Design review of the part built by this model. Coordinates are the model's own, in mm. A direction names the side the tool comes from. Give positions to 0.01 mm unless a question says otherwise; leave off trailing zeros. Loops run counter-clockwise (first coordinate to the right, second up) from the corner with the lowest first, then second, coordinate; pieces in that order, holes last.
from build123d import *

# Parameters (mm, degrees)
SKETCH1_R           = 1.651
BOSS_EXTRUDE1_DEPTH = 6.35
SKETCH2_W           = 12.7
SKETCH2_H           = 3.175
CUT_EXTRUDE7_DEPTH  = 8.89
FILLET2_R           = 1.27
SKETCH4_W           = 3.175
SKETCH4_H           = 19.05
CUT_EXTRUDE8_DEPTH  = 192.82600491
FILLET3_R           = 1.27
SKETCH5_R           = 3.175
CUT_EXTRUDE9_DEPTH  = 2.54


with BuildPart() as part:
    # Sketch1 → Boss-Extrude1 (new body)
    with BuildSketch(Plane(origin=(0, 0, 0), x_dir=(1, 0, 0), z_dir=(0, 1, 0))):
        Polygon((75.155177047, 61.997896552), (75.155177047, 11.997896552), (91.919177047, 11.997896552), (91.919177047, 20.379896552), (83.537177047, 20.379896552), (83.537177047, 53.615896552), (173.037829354, 53.615896552), (173.037829354, 20.379896552), (164.655829354, 20.379896552), (164.655829354, 11.997896552), (181.419829354, 11.997896552), (181.419829354, 61.997896552), align=None)
        with Locations(Location((80.3721812, 16.064784874, 0), (0, 0, 270))):
            Circle(SKETCH1_R, mode=Mode.SUBTRACT)
        with Locations(Location((80.3721812, 57.93100823, 0), (0, 0, 270))):
            Circle(SKETCH1_R, mode=Mode.SUBTRACT)
        with Locations(Location((88.7874552, 16.064784874, 0), (0, 0, 270))):
            Circle(SKETCH1_R, mode=Mode.SUBTRACT)
        with Locations(Location((167.7875512, 57.93100823, 0), (0, 0, 270))):
            Circle(SKETCH1_R, mode=Mode.SUBTRACT)
        with Locations(Location((88.7874552, 57.93100823, 0), (0, 0, 270))):
            Circle(SKETCH1_R, mode=Mode.SUBTRACT)
        with Locations(Location((176.2028252, 57.93100823, 0), (0, 0, 270))):
            Circle(SKETCH1_R, mode=Mode.SUBTRACT)
        with Locations(Location((176.2028252, 16.064784874, 0), (0, 0, 270))):
            Circle(SKETCH1_R, mode=Mode.SUBTRACT)
        with Locations(Location((167.7875512, 16.064784874, 0), (0, 0, 270))):
            Circle(SKETCH1_R, mode=Mode.SUBTRACT)
    extrude(amount=BOSS_EXTRUDE1_DEPTH)

    # Sketch2 → Cut-Extrude7 (cut)
    with BuildSketch(Plane(origin=(181.419829354, 0, 0), x_dir=(0, 0, -1), z_dir=(1, 0, 0))):
        with Locations((43.747896552, 4.7625)):
            Rectangle(SKETCH2_W, SKETCH2_H)
    extrude(amount=-CUT_EXTRUDE7_DEPTH, mode=Mode.SUBTRACT)

    # Fillet2
    fillet2_edges = [part.edges().sort_by_distance(p)[0] for p in [
        (177.228829354, 6.35, -37.397896552),
        (177.228829354, 6.35, -50.097896552),
        (177.228829354, 3.175, -50.097896552),
        (177.228829354, 3.175, -37.397896552),
    ]]
    fillet(fillet2_edges, radius=FILLET2_R)

    # Sketch4 → Cut-Extrude8 (cut, through all)
    with BuildSketch(Plane(origin=(0, 6.35, 0), x_dir=(1, 0, 0), z_dir=(0, 1, 0))):
        with Locations((81.949677047, 29.904896552)):
            Rectangle(SKETCH4_W, SKETCH4_H)
    extrude(amount=-CUT_EXTRUDE8_DEPTH, mode=Mode.SUBTRACT)

    # Fillet3
    fillet3_edges = [part.edges().sort_by_distance(p)[0] for p in [
        (83.537177047, 3.175, -39.429896552),
        (80.362177047, 3.175, -20.379896552),
        (80.362177047, 3.175, -39.429896552),
    ]]
    fillet(fillet3_edges, radius=FILLET3_R)

    # Sketch5 → Cut-Extrude9 (cut)
    with BuildSketch(Plane.XZ):
        with Locations((88.7874552, -16.064784874)):
            Circle(SKETCH5_R)
        with Locations(Location((88.7874552, -57.93100823, 0), (0, 0, 270))):
            Circle(SKETCH5_R)
        with Locations(Location((167.7875512, -57.93100823, 0), (0, 0, 270))):
            Circle(SKETCH5_R)
        with Locations((167.7875512, -16.064784874)):
            Circle(SKETCH5_R)
    extrude(amount=-CUT_EXTRUDE9_DEPTH, mode=Mode.SUBTRACT)


solid = part.part
Q1. Take a section at C-C (y = 1.25). Give the boundary of the cut face in (x, z) (3 decimals).
Results:
outline: (75.155, -61.998) - (181.42, -61.998) - (181.42, -11.998) - (164.656, -11.998) - (164.656, -15.542) arc R3.175 cw (long way) to (164.656, -16.587) - (164.656, -20.38) - (173.038, -20.38) - (173.038, -53.616) - (83.537, -53.616) - (83.537, -40.7) arc R1.27 ccw to (82.267, -39.43) - (81.632, -39.43) arc R1.27 cw to (80.362, -38.16) - (80.362, -21.65) arc R1.27 cw to (81.632, -20.38) - (91.919, -20.38) - (91.919, -16.587) arc R3.175 cw (long way) to (91.919, -15.542) - (91.919, -11.998) - (75.155, -11.998) - close; hole circle Ø3.302 at (80.372, -57.931); hole circle Ø3.302 at (80.372, -16.065); hole circle Ø6.35 at (88.787, -57.931); hole circle Ø6.35 at (167.788, -57.931); hole circle Ø3.302 at (176.203, -57.931); hole circle Ø3.302 at (176.203, -16.065)
Q2. Draft analysis for pull direction Z (two halves, no side actions). For faces 1 (the face through (173, 3, -11.998)), 2 (the face through (129, 3, -61.998)), 3 (the face through (170.96, 1.25, -16.2)), 4 (the face through (91.919, 3, -16)), state which applies: pulls with the +Z half, pulls with the -Z half, needs draft (parallel to the pull), parting line crosses it, or undercut.
Results:
face 1: pulls with the +Z half
face 2: pulls with the -Z half
face 3: undercut
face 4: needs draft
Q3. Take a section at D-D (x = 125.5). Give the boundary of the cut face in (y, z).
Results:
outline: (0, -62) - (6.35, -62) - (6.35, -53.62) - (0, -53.62) - close
Q4. Tool access review of faces 5 (the face through (128, 3, -53.616)), 6 (the face through (177, 3.175, -44)), 7 (the face through (166, 2.54, -59)): name each direction out of +Z, -Z, +X, -X, +Y, -Y from which nothing blocks a thin tool from reaching the whole face with its end or side.
Results:
face 5: +Y, -Y
face 6: +X, +Y
face 7: -Y
Q5. Insertion check: pin 1 (2 mm diameter, centred on x = 176.2, z = -57.93, fed in from +Y); pin 2 (9 mm diameter, centred on x = 177, z = -44.5, fed in from +Y); pin 3 (5 mm diameter, centred on x = 88.79, z = -16.06, fed in from +Y); pin 4 (1.9 mm diameter, centred on x = 89.5, z = -57, fed in from -Y). Each pin has a flat end and moves straight along its axis. Give the tip position at first contact, or say it passes through.
Results:
pin 1: passes through
pin 2: stops at y = 3.19
pin 3: stops at y = 6.35
pin 4: stops at y = 2.54
Q6. Take a section at A-A (z = -52.5). Give the boundary of the cut face in (x, y), plus the area to 3 significant figures.
Results:
outline: (75.16, 0) - (83.54, 0) - (83.54, 6.35) - (75.16, 6.35) - close; (173.04, 0) - (181.42, 0) - (181.42, 6.35) - (173.04, 6.35) - close
area: 106 mm2
Q7. Wall thickness on line 1 (X direction, y = 6, z = -58); line 2 (X direction, y = 5.5, z = -37); line 3 (X direction, y = 1.5, z = -50.5): over which ranges is each line inside the solid? List them lowest first.
Results:
line 1: x = 75.16 to 78.72, 82.02 to 87.14, 90.44 to 166.14, 169.44 to 174.55, 177.85 to 181.42
line 2: x = 75.16 to 80.36, 173.04 to 181.42
line 3: x = 75.16 to 83.54, 173.04 to 181.42
Q8. Take a section at B-B (z = -44). Give the boundary of the cut face in (x, y) (3 decimals), plus the area to 3 significant figures.
Results:
outline: (75.155, 0) - (83.537, 0) - (83.537, 6.35) - (75.155, 6.35) - close; (173.038, 0) - (181.42, 0) - (181.42, 3.175) - (173.038, 3.175) - close
area: 79.8 mm2
